Study the drawing (mm; zero at the part's minimum x, y, z) and answer. A direction names the side the tool comes from. Coordinates: 2 decimals unless noted, no trailing zeros. Loops run counter-clockwise (first coordinate to the right, second up) from the corner with the lowest first, then second, coordinate; pieces in that order, holes last.
Q1. Section A-A (x = 4.05) is taken. Give the vertices of the cut face in (y, z), then the cut area to 3 significant figures.
Q2. Section D-D (y = 14.5) is taken. Give the vertices of the cut face in (x, z), then the cut area to 3 significant figures.
Q3. Which of the six approach directions +Z, -Z, +X, -X, +Y, -Y give full straight-line access (tool end or side, diameter ignored) to the marked faces 5, 6 and 7?
Q4. Section B-B (z = 3.5) is taken. Give the vertices of the cut face in (x, y).
Q5. Straight lines are drawn through the part: line 1 (X direction, y = 9.95, z = 2.4); line 2 (X direction, y = 9.95, z = 0.95); line 3 (Y direction, x = 31, z = 1.5). For each, find the intervals that lie inside material, in ascending order.
Q6. Section C-C (y = 9.95) is taken. Give the vertices of the cut face in (x, z), then the cut area to 3 significant figures.
Q7. Flat-ended cylindrical pins translate along their axes: P1, Ø2.5, axis at x = 26.5, z = 2, coming from the -Y side; P2, Ø4.5, axis at y = 4.5, z = 2.5, coming from the -X side; P3, Ø3.5, axis at x = 50.5, y = 8, coming from the +Z side. Find the tip coordinate at first contact, or state that the pin passes through.
Q8. The mould has two halves that part along Y. Classify the marked faces 1, 2, 3 and 4: pulls with the +Y half, pulls with the -Y half, needs draft (parallel to the pull), parting line crosses it, or undercut.
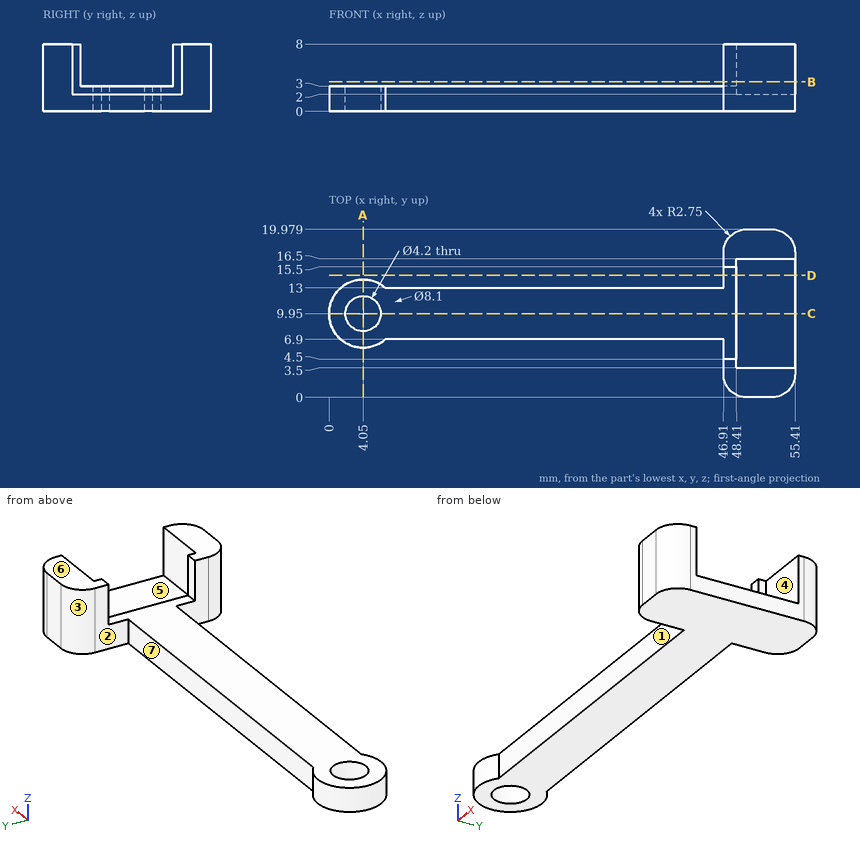
Numbers:
1. outline: (5.9, 0) - (7.85, 0) - (7.85, 3) - (5.9, 3) - close; (12.05, 0) - (14, 0) - (14, 3) - (12.05, 3) - close
1. area: 11.7 mm2
2. outline: (46.91, 0) - (55.41, 0) - (55.41, 2) - (48.41, 2) - (48.41, 3) - (46.91, 3) - close
2. area: 18.5 mm2
3. face 5: +Z, +X
3. face 6: +Z, +X, -X, +Y, -Y
3. face 7: +Z, -Z, +Y
4. outline: (46.91, 2.75) arc R2.75 ccw to (49.66, 0) - (52.66, 0) arc R2.75 ccw to (55.41, 2.75) - (55.41, 3.5) - (48.41, 3.5) - (48.41, 4.5) - (46.91, 4.5) - close; (46.91, 15.5) - (48.41, 15.5) - (48.41, 16.5) - (55.41, 16.5) - (55.41, 17.23) arc R2.75 ccw to (52.66, 19.98) - (49.66, 19.98) arc R2.75 ccw to (46.91, 17.23) - close
5. line 1: x = 0 to 1.95, 6.15 to 48.41
5. line 2: x = 0 to 1.95, 6.15 to 55.41
5. line 3: y = 6.9 to 13
6. outline: (0, 0) - (1.95, 0) - (1.95, 3) - (0, 3) - close; (6.15, 0) - (55.41, 0) - (55.41, 2) - (48.41, 2) - (48.41, 3) - (6.15, 3) - close
6. area: 147 mm2
7. P1: stops at y = 6.9
7. P2: stops at x = 1.57
7. P3: stops at z = 2
8. face 1: pulls with the -Y half
8. face 2: needs draft
8. face 3: pulls with the +Y half
8. face 4: undercut
